Input: dimensioned drawing with shaded views. Units: mm. Origin: part minimum x, y, z. Give positions to 0.01 mm unless a question says otherwise; leave off trailing zeros. Write each loop counter-clockwise with the first axis right and the second up, starting at its lowest first coordinate (ties: lowest second). Pieces come first, ordered by that corner, then holes.
Q1. Line query: line 1 (Z direction, x = 58, y = 28); line 2 (Z direction, x = 71, y = 202.5); line 3 (X direction, y = 264, z = 10). Output: solid intervals per line, ascending.
Q2. Section A-A (y = 33.5). Return the cut outline in (x, z).
Q3. Pin query (flat end, axial travel): pin 1 Ø6 at (y, z) = (175.5, 25) entering from +X (1 decimal); pin 2 Ø5 at (y, z) = (154.5, 29.5) entering from -X; pin 3 Ø5 at (y, z) = (191.5, 7.5) entering from +X; pin 4 Ø12 at (x, y) = (50.5, 63.5) entering from +Z. Return the tip coordinate at first contact, or that it passes through.
Q4. Section B-B (z = 7.5). Return the cut outline in (x, y).
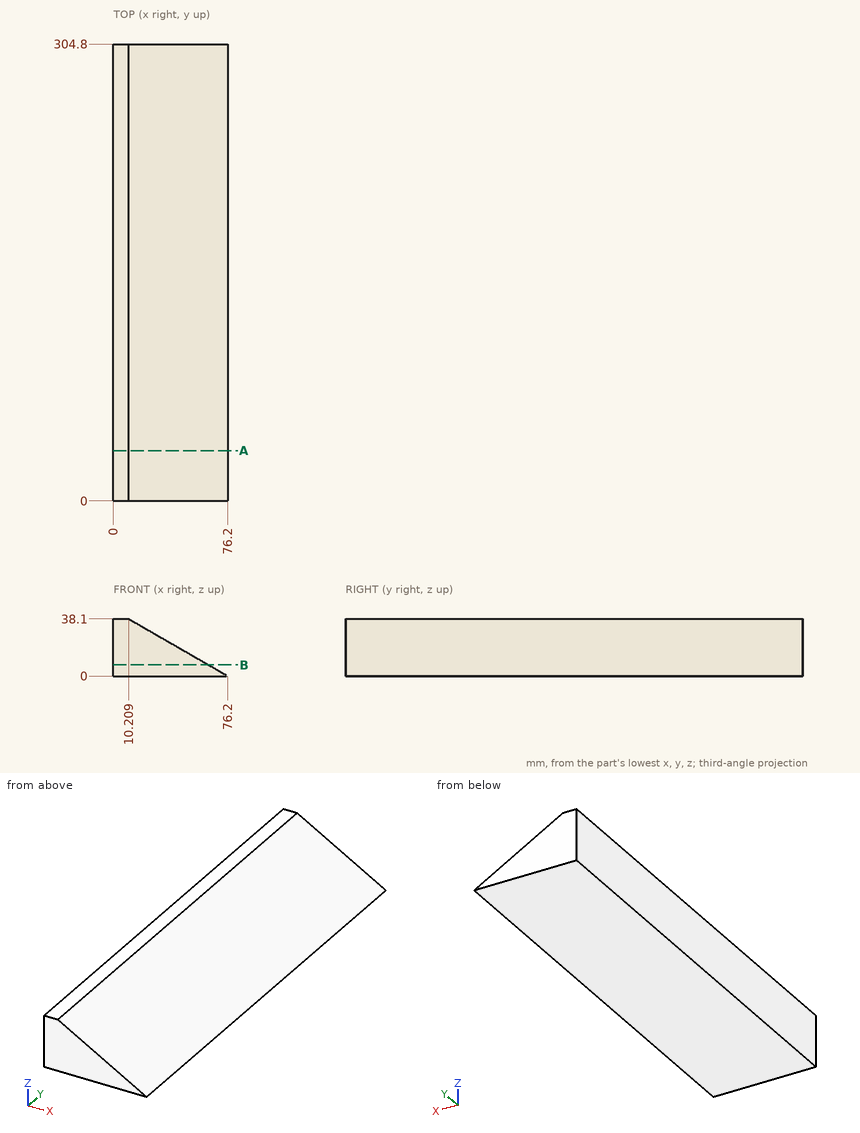
Computed:
1. line 1: z = 0 to 10.51
1. line 2: z = 0 to 3
1. line 3: x = 0 to 58.88
2. outline: (0, 0) - (76.2, 0) - (10.21, 38.1) - (0, 38.1) - close
3. pin 1: stops at x = 38.1
3. pin 2: stops at x = 0
3. pin 3: stops at x = 67.54
3. pin 4: stops at z = 18.3
4. outline: (0, 0) - (63.21, 0) - (63.21, 304.8) - (0, 304.8) - close
